```python
from build123d import *

# Parameters (mm, degrees)
SKETCH_1_R               = 35
EXTRUDE_1_DEPTH          = 23
SKETCH_2_R               = 1.9
EXTRUDE_2_DEPTH          = 11
SKETCH_4_W               = 3.8
SKETCH_4_H               = 34.948390521
EXTRUDE_6_DEPTH          = 3
PATTERN_CIRCULAR_1_COUNT = 12
CUT_EXTRUDE_3_DEPTH      = 4
PATTERN_CIRCULAR_2_COUNT = 12


with BuildPart() as part:
    # Эскиз1 → Бобышка-Вытянуть1 (new body)
    with BuildSketch(Plane(origin=(0, 0, 0), x_dir=(1, 0, 0), z_dir=(0, 1, 0))):
        Circle(SKETCH_1_R)
    extrude(amount=EXTRUDE_1_DEPTH)

    # Эскиз2 → Бобышка-Вытянуть2 (add)
    with BuildSketch(Plane(origin=(0, 23, 0), x_dir=(1, 0, 0), z_dir=(0, 1, 0))):
        Circle(SKETCH_2_R)
    extrude(amount=EXTRUDE_2_DEPTH)

    # Эскиз4 → Бобышка-Вытянуть6 (add)
    with BuildSketch(Plane(origin=(0, 23, 0), x_dir=(1, 0, 0), z_dir=(0, 1, 0))):
        with Locations((0, 17.474195261)):
            Rectangle(SKETCH_4_W, SKETCH_4_H)
    extrude_6 = extrude(amount=EXTRUDE_6_DEPTH)

    # Круговой массив1: Бобышка-Вытянуть6 ×12 about axis
    pattern_circular_1_axis = Axis((0, 0, 0), (0, 1, 0))
    for i in range(1, PATTERN_CIRCULAR_1_COUNT):
        add(extrude_6.rotate(pattern_circular_1_axis, i * 360 / PATTERN_CIRCULAR_1_COUNT))

    # Эскиз12 → Вырез-Вытянуть3 (cut)
    with BuildSketch(Plane(origin=(-0.95, 0, 1.645448267), x_dir=(0.866025404, 0, 0.5), z_dir=(-0.5, 0, 0.866025404))):
        with BuildLine():
            add(Edge.make_bspline(
                [(-34.948390521, 23), (-21.115111168, 25.388771588), (-7.090896534, 26)],
                knots=[0, 0, 0, 1, 1, 1], degree=2))
            Line((-7.090896534, 26), (-34.948390521, 26))
            Line((-34.948390521, 26), (-34.948390521, 23))
        make_face()
    cut_extrude_3 = extrude(amount=-CUT_EXTRUDE_3_DEPTH, mode=Mode.SUBTRACT)

    # Круговой массив2: Вырез-Вытянуть3 ×12 about axis
    pattern_circular_2_axis = Axis((0, 0, 0), (0, -1, 0))
    for i in range(1, PATTERN_CIRCULAR_2_COUNT):
        add(cut_extrude_3.rotate(pattern_circular_2_axis, i * 360 / PATTERN_CIRCULAR_2_COUNT), mode=Mode.SUBTRACT)


solid = part.part
```
Input: part model. Units: mm. Frame: model coordinates. A direction names the side the tool comes from. Coordinates: 2 decimals unless noted, no trailing zeros. Loops run counter-clockwise (first coordinate to the right, second up) from the corner with the lowest first, then second, coordinate; pieces in that order, holes last. Notation, with made-up numbers: (32, 31) - (50, 31) arc R26 ccw to (50, 69) - close; hole circle Ø8 at (47, 72). An arc over 180 degrees is marked (long way). Answer in a Markdown table with one row per item.
(1) Mould query, pull axis X, two halves, no side actions, for faces 3 (the face through (14.4, 24.15, -10.51)), 4 (the face through (-24, 23, 7)). Classes: pulls with the +X half, pulls with the -X half, needs draft (parallel to the pull), parting line crosses it, or undercut.
Model answer:
| item | result |
|---|---|
| face 3 | undercut |
| face 4 | needs draft |
(2) Material intervals for L1, parallel to Y at x = 12.5, z = -3; L2, parallel to Y at x = 13, z = 9.5; L3, parallel to X at y = 4, z = 10, sorted ascending. Write a range as from..to.
Model answer:
| item | result |
|---|---|
| L1 | y = 0..23 |
| L2 | y = 0..25.43 |
| L3 | x = -33.54..33.54 |
(3) Cut plane B-B on y = 30. Output: boundary loops of the cut face in (x, z), plus the area to 3 significant figures.
Model answer:
| item | result |
|---|---|
| outline | circle Ø3.8 at (0, 0) |
| area | 11.3 mm² |
(4) Set-up query: faces 1 (the face through (-17, 23, 18)), 2 (the face through (-7, 23, -24)). Return all of +Z, -Z, +X, -X, +Y, -Y with unobstructed straight access to the full face (end or side cutting, diameter ignored); none if empty.
Model answer:
| item | result |
|---|---|
| face 1 | +Y |
| face 2 | -Z, +Y |
(5) Cut plane A-A on y = 7.5. Output: boundary loops of the cut face in (x, z), plus the area to 3 significant figures.
Model answer:
| item | result |
|---|---|
| outline | circle Ø70 at (0, 0) |
| area | 3,850 mm² |
(6) Pin query (flat end, axial travel): P1, Ø1, axis at y = 27, z = 10.5, coming from the +X side; P2, Ø2.5, axis at y = 25, z = -21.5, coming from the +X side; P3, Ø15.5, axis at x = 21, z = 12, coming from the +Y side; P4, Ø2, axis at x = -30.5, z = 17.5, coming from the +Y side. Return the tip coordinate at first contact, or that it passes through.
Model answer:
| item | result |
|---|---|
| P1 | passes through |
| P2 | stops at x = 15.17 |
| P3 | stops at y = 25.39 |
| P4 | stops at y = 23.13 |
